Design review of the part built by this model. Coordinates are the model's own, in mm. Coordinates: 2 decimals unless noted, no trailing zeros. Loops run counter-clockwise (first coordinate to the right, second up) from the corner with the lowest first, then second, coordinate; pieces in that order, holes last.
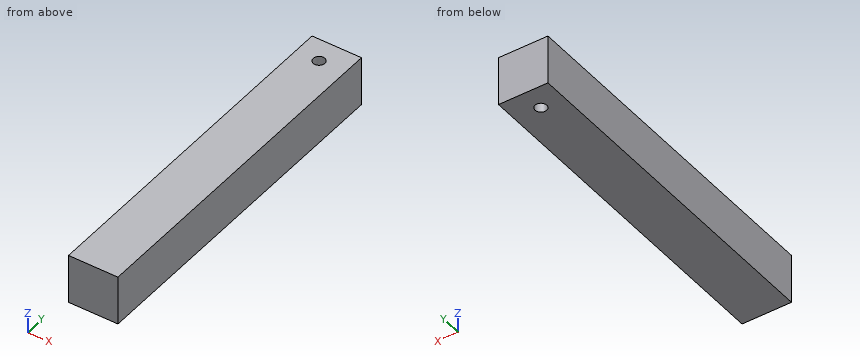
from build123d import *

# Parameters (mm, degrees)
SKETCH1_W           = 21.59
SKETCH1_H           = 21.59
BOSS_EXTRUDE1_DEPTH = 152.4
SKETCH2_R           = 2.54
CUT_EXTRUDE1_DEPTH  = 26.67


with BuildPart() as part:
    # Sketch1 → Boss-Extrude1 (new body)
    with BuildSketch(Plane(origin=(0, 0, 0), x_dir=(1, 0, 0), z_dir=(0, 1, 0))):
        with Locations((10.795, -10.795)):
            Rectangle(SKETCH1_W, SKETCH1_H)
    extrude(amount=BOSS_EXTRUDE1_DEPTH)

    # Sketch2 → Cut-Extrude1 (cut)
    with BuildSketch(Plane.XY):
        with Locations(Location((10.16, 142.24, 0), (0, 0, 180))):
            Circle(SKETCH2_R)
    extrude(amount=CUT_EXTRUDE1_DEPTH, mode=Mode.SUBTRACT)


solid = part.part
Q1. Take a section at A-A, the plane x = 10.16. Write out the cut boundary in (y, z), then the cut area to 3 significant figures.
Q2. Take a section at B-B, the plane y = 142.24. Write out the cut boundary in (x, z), then the cut area to 3 significant figures.
Q3. For line 1 (X direction, y = 142.24, z = 11); line 2 (Y direction, x = 10.16, z = 12.5); line 3 (Y direction, x = 12, z = 18.5), list the stretches that pass through material, from the lowest coordinate up.
Entries:
1. outline: (0, 0) - (139.7, 0) - (139.7, 21.59) - (0, 21.59) - close; (144.78, 0) - (152.4, 0) - (152.4, 21.59) - (144.78, 21.59) - close
1. area: 3,180 mm2
2. outline: (0, 0) - (7.62, 0) - (7.62, 21.59) - (0, 21.59) - close; (12.7, 0) - (21.59, 0) - (21.59, 21.59) - (12.7, 21.59) - close
2. area: 356 mm2
3. line 1: x = 0 to 7.62, 12.7 to 21.59
3. line 2: y = 0 to 139.7, 144.78 to 152.4
3. line 3: y = 0 to 140.49, 143.99 to 152.4
